from build123d import *

# Parameters (mm, degrees)
PAD002_DEPTH         = 40
SKETCH005_R          = 2
POCKET002_DEPTH      = 11.42
POCKET002_DEPTH_BACK = 11.42
FILLET003_R          = 2


with BuildPart() as part:
    # Sketch004 → Pad002 (new body)
    with BuildSketch(Plane.XY):
        with BuildLine():
            ThreePointArc((-7.404873, 11.419), (-10.165124, 0), (-7.404873, -11.419))
            Line((-18.540205, -8), (-7.404873, -11.419))
            Line((-35.165124, -8), (-18.540205, -8))
            Line((-35.165124, 8), (-35.165124, -8))
            Line((-18.540205, 8), (-35.165124, 8))
            Line((-7.404873, 11.419), (-18.540205, 8))
        make_face()
    extrude(amount=PAD002_DEPTH)

    # Sketch005 → Pocket002 (cut, two sides)
    with BuildSketch(Plane.XZ) as pocket002_sk:
        with Locations((-27, 30)):
            Circle(SKETCH005_R)
        with Locations((-27, 10)):
            Circle(SKETCH005_R)
    extrude(amount=-POCKET002_DEPTH, mode=Mode.SUBTRACT)
    extrude(pocket002_sk.sketch, amount=POCKET002_DEPTH_BACK, mode=Mode.SUBTRACT)

    # Fillet003
    fillet003_edges = [part.edges().sort_by_distance(p)[0] for p in [
        (-35.165124, 0, 40),
        (-35.165124, 0, 0),
    ]]
    fillet(fillet003_edges, radius=FILLET003_R)


with BuildPart() as part_1:
    # Body002 placement: moved
    add(part.part.moved(Location((-30, 0, 0))))


solid = part_1.part
Work out the finished part from the listing and answer in its coordinate system (mm). A direction names the side the tool comes from. Round coordinates to 2 decimals unless told otherwise and drop trailing zeros. Write each loop counter-clockwise with the first axis right and the second up, starting at its lowest first coordinate (ties: lowest second). Pieces come first, ordered by that corner, then holes. Notation, with made-up numbers: M 9.5,17 L 62.5,17 A25 ccw 62.5,42 Z; hole C -5.75,-20 d8. An arc over 180 degrees is marked long. Use a Markdown table: item, result.
1) Flat-ended cylindrical pins translate along their axes: pin 1 (3.5 mm diameter, centred on x = -57, z = 30, fed in from +Y); pin 2 (4.5 mm diameter, centred on x = -57, z = 10, fed in from +Y); pin 3 (2 mm diameter, centred on x = -44, z = 34, fed in from +Y); pin 4 (8.5 mm diameter, centred on x = -58, z = 18, fed in from -Y). Find the tip coordinate at first contact, or state that the pin passes through.
Taken from the geometry:
| item | result |
|---|---|
| pin 1 | passes through |
| pin 2 | stops at y = 8 |
| pin 3 | stops at y = 9.7 |
| pin 4 | stops at y = -8 |
2) The part is cut by section D-D on z = 37. Give the vertices of the cut face in (x, y), plus the area to 3 significant figures.
Taken from the geometry:
| item | result |
|---|---|
| outline | M -65.17,-8 L -48.54,-8 L -37.4,-11.42 A25 cw -37.4,11.42 L -48.54,8 L -65.17,8 Z |
| area | 440 mm2 |
3) The part is cut by section A-A on x = -57. Give the vertices of the cut face in (y, z).
Taken from the geometry:
| item | result |
|---|---|
| outline | M -8,0 L 8,0 L 8,8 L -8,8 Z; M -8,12 L 8,12 L 8,28 L -8,28 Z; M -8,32 L 8,32 L 8,40 L -8,40 Z |
4) Determine the mould class of faces 1 (the face through (-56.077, -0.112, 28.226)), 2 (the face through (-50, 0, 0)), 3 (the face through (-65.165, 0, 20)) for opening direction Z: pulls with the +Z half, pulls with the -Z half, needs draft (parallel to the pull), parting line crosses it, or undercut.
Taken from the geometry:
| item | result |
|---|---|
| face 1 | undercut |
| face 2 | pulls with the -Z half |
| face 3 | needs draft |
5) The part is cut by section C-C on y = 7.5. Give the vertices of the cut face in (x, z), plus the area to 3 significant figures.
Taken from the geometry:
| item | result |
|---|---|
| outline | M -65.17,2 A2 ccw -63.17,0 L -39.01,0 L -39.01,40 L -63.17,40 A2 ccw -65.17,38 Z; hole C -57,10 d4; hole C -57,30 d4 |
| area | 1,020 mm2 |
6) The part is cut by section B-B on z = 30. Give the vertices of the cut face in (x, y), plus the area to 3 significant figures.
Taken from the geometry:
| item | result |
|---|---|
| outline | M -65.17,-8 L -59,-8 L -59,8 L -65.17,8 Z; M -55,-8 L -48.54,-8 L -37.4,-11.42 A25 cw -37.4,11.42 L -48.54,8 L -55,8 Z |
| area | 376 mm2 |
7) Which of the six approach directions +Z, -Z, +X, -X, +Y, -Y give full straight-line access (tool end or side, diameter ignored) to faces 4 (the face through (-57, -8, 20)), 5 (the face through (-64.595, -0.112, 0.601)), 6 (the face through (-57, 8, 20))?
Taken from the geometry:
| item | result |
|---|---|
| face 4 | +Z, -Z, -X, -Y |
| face 5 | -Z, -X, +Y, -Y |
| face 6 | +Z, -Z, -X, +Y |
8) Consider line 1 (Z direction, x = -57, y = -2); line 2 (X direction, y = 0.25, z = 30); line 3 (Z direction, x = -58.25, y = 6.25). Determine where each line is inside the solid, lowest interval first. Write a range as [from, to].
Taken from the geometry:
| item | result |
|---|---|
| line 1 | z = [0, 8], [12, 28], [32, 40] |
| line 2 | x = [-65.17, -59], [-55, -40.16] |
| line 3 | z = [0, 8.44], [11.56, 28.44], [31.56, 40] |
